Autodesk Inventor part; units mm, degrees
ref_plane "YZ Plane" through (0, 0, 0) normal (1, 0, 0) x (0, 1, 0)
ref_plane "XZ Plane" through (0, 0, 0) normal (0, 1, 0) x (-1, 0, 0)
ref_plane "XY Plane" through (0, 0, 0) normal (0, 0, 1) x (1, 0, 0)
sketch "Sketch1" plane through (0, 0, 0) normal (0, 0, 1) x (1, 0, 0)
  circle A0 centre (10, 11.5) radius 1.6
  line L0 (0, 0) -> (20.0001, 0)
  line L1 (0, 0) -> (0, 3)
  line L2 (20.0001, 0) -> (20.0001, 3)
  line L3 (0, 3) -> (16, 3) construction
  line L4 (20.0001, 3) -> (36.0001, 3) construction
  arc A1 (14.3301, 14) -> (5.6699, 14) centre (10, 11.5) ccw
  line L5 (10, 11.5) -> (5.6699, 14) construction
  line L6 (10, 11.5) -> (14.3301, 14) construction
  line L7 (5.6699, 14) -> (0, 3)
  line L8 (14.3301, 14) -> (20.0001, 3)
  dimension "d17" = 3
  dimension "d18" = 3
  dimension "d19" = 11.5
  dimension "d23" = 90
  dimension "d24" = 90
  dimension "d25" = 10
  dimension "d31" = 5
  dimension "d32" = 120
  dimension "d33" = 14
sketch "Sketch3" plane through (0, 0, 0) normal (0, 0, 1) x (1, 0, 0)
  point P0 (0, 0)
extrude "Extrusion1" add sketch "Sketch1" along normal blind 4.2
sketch "Sketch4" plane through (0, 0, 4.2) normal (0, 0, 1) x (1, 0, 0)
  line L0 (0, 3) -> (0, 0)
  line L1 (20.0001, 0) -> (20.0001, 3)
  line L2 (0, 0) -> (20.0001, 0)
  line L3 (20.0001, 0) -> (20.0001, 3)
  line L4 (3.884, 22.9404) -> (-0.9789, 3.2417)
  line L5 (20.0001, 3) -> (0, 3)
  line L6 (0, 3) -> (0, 0)
extrude "Extrusion2" add sketch "Sketch4" along normal blind 4.2
sketch "Sketch5" plane through (0, 0, 0) normal (0, -1, 0) x (1, 0, 0)
  circle A0 centre (5, 4.8) radius 0.5
  circle A1 centre (15, 4.8) radius 0.5
  line L0 (0, 0) -> (20.0001, 0)
  dimension "d13" = 1
  dimension "d14" = 1
  dimension "d38" = 4.8
  dimension "d39" = 4.8
extrude "Extrusion3" cut sketch "Sketch5" against normal blind 5.5
sketch "Sketch6" plane through (0, 3, 8.4) normal (0, 1, 0) x (1, 0, 0)
  circle A0 centre (5, 3.6) radius 0.5
  circle A1 centre (5, 3.6) radius 3
  circle A2 centre (15, 3.6) radius 0.5
  circle A3 centre (15, 3.6) radius 3
  line L0 (0, 8.4) -> (20.0001, 8.4)
  dimension "d34" = 6
  dimension "d35" = 6
  dimension "d40" = 4.8
  dimension "d41" = 4.8
extrude "Extrusion4" cut sketch "Sketch6" along normal up to next
properties part number "lower_deck_shaft_mount"
Model file for the job. Use its own axes, mm. A direction names the side the tool comes from. Coordinates: 2 decimals unless noted, no trailing zeros. Order: outer loops, then holes, each group sorted by start corner. A loop starts at its lowest first (then second) coordinate and runs counter-clockwise, first axis right, second up. Notation, with made-up numbers: (43.25, 78) -> (65.25, 78) arc R13 ccw to (65.25, 93) -> close; hole circle Ø9 at (5, 14). An arc over 180 degrees is marked (long way). Return JSON: item names as keys, results as strings. Group by question number.
Item 1: Flat gauge pins, fed straight in: P1, Ø2, axis at y = 14.5, z = 2, coming from the +X side; P2, Ø3, axis at x = 10.5, y = 9.5, coming from the +Z side; P3, Ø1.5, axis at y = 12.5, z = 1.5, coming from the -X side. Where does each tip first touch, or does it go through?
Item 2: Saw through at C-C on z = 3. Write the cut outline in (x, y).
Item 3: Wall check: line 1 along Y through (x, z) = (10, 2.3); line 2 along Z through (x, y) = (5, 0.9); line 3 along Y through (x, z) = (10.5, 7.5). Give the ranges that are in metal, low to high. Write a range as [from, to].
Item 4: Saw through at B-B on y = 11.5. Write the cut outline in (x, z), then the cut area to 3 significant figures.
Item 5: Saw through at A-A on x = 10. Write the cut outline in (y, z).
Item 6: Pull direction Z, two halves, no side cores. Call faces 4 (the cylindrical face through (14.046, 7.986, 1.956)), 5 (the cylindrical face through (8.4, 11.43, 2.07)), 6 (the cylindrical face through (14.892, 1.479, 4.312)): pulls with the +Z half, pulls with the -Z half, needs draft (parallel to the pull), parting line crosses it, or undercut.
Item 7: Tool access for faces 1 (the flat face through (9.5, 9.8, 4.2)), 2 (the flat face through (10, 3, 6)), 3 (the flat face through (10, 2, 8.4)): list every direction of +Z, -Z, +X, -X, +Y, -Y with a clear straight run to the whole face (end or side of a thin tool).
Item 8: Saw through at D-D on y = 13.5. Write the cut outline in (x, z).
Values found:
{
 "1": {"P1": "stops at x = 14.58", "P2": "stops at z = 4.2", "P3": "stops at x = 4.51"},
 "2": {"outline": "(0, 0) -> (20, 0) -> (20, 3) -> (17.4, 8.04) -> (17.4, 3) -> (12.6, 3) -> (12.6, 15.77) arc R5 ccw to (7.4, 15.77) -> (7.4, 3) -> (2.6, 3) -> (2.6, 8.04) -> (0, 3) -> close; hole circle Ø3.2 at (10, 11.5)"},
 "3": {"line 1": "y = [0, 9.9], [13.1, 16.5]", "line 2": "z = [0, 4.3], [5.3, 8.4]", "line 3": "y = [0, 3]"},
 "4": {"outline": "(4.38, 0) -> (8.4, 0) -> (8.4, 4.2) -> (7.94, 4.2) arc R3 cw to (4.38, 1.86) -> close; (11.6, 0) -> (15.62, 0) -> (15.62, 1.86) arc R3 cw to (12.06, 4.2) -> (11.6, 4.2) -> close", "area": "20.3 mm2"},
 "5": {"outline": "(0, 0) -> (9.9, 0) -> (9.9, 4.2) -> (3, 4.2) -> (3, 8.4) -> (0, 8.4) -> close; (13.1, 0) -> (16.5, 0) -> (16.5, 4.2) -> (13.1, 4.2) -> close"},
 "6": {"face 4": "pulls with the +Z half", "face 5": "needs draft", "face 6": "undercut"},
 "7": {"face 1": "+Z, +X, -X, +Y", "face 2": "+Z, +Y", "face 3": "+Z, +X, -X, +Y, -Y"},
 "8": {"outline": "(5.41, 0) -> (14.59, 0) -> (14.59, 1.83) arc R3 cw to (12.06, 4.2) -> (7.94, 4.2) arc R3 cw to (5.41, 1.83) -> close"}
}
